Input: part model. Units: mm. Frame: model coordinates. A direction names the side the tool comes from. Coordinates: 2 decimals unless noted, no trailing zeros. Loops run counter-clockwise (first coordinate to the right, second up) from the corner with the lowest first, then second, coordinate; pieces in that order, holes last. Notation, with made-up numbers: (-39, 63.25) - (-4, 63.25) arc R9 ccw to (-4, 70.25) - close; hole circle Ø8 at (-3, -34.5). An arc over 180 degrees is marked (long way). Write item = value, one per line. Start each with the question number.
from build123d import *

# Parameters (mm, degrees)
F1_DEPTH    = 76.2
F2_T1_DEPTH = 369.824
F2_T3_DEPTH = 369.824


# Not quite as in the source:
# - a fillet or chamfer that OpenCascade refuses, or shapes differently, is made with other operations: its cross-section is extruded or revolved along the edge and cut away or added


with BuildPart() as f1:
    # F0 (on Right) → F1 (new body, symmetric)
    with BuildSketch(Plane.YZ):
        with BuildLine():
            Line((-304.8, 0), (0, 0))
            Line((0, 0), (304.8, 0))
            ThreePointArc((304.8, 0), (353.0430518596, 9.3618295777), (390.9983313803, 40.5777335736))
            Line((390.9983313803, 40.5777335736), (381.1075556217, 50.8))
            ThreePointArc((381.1075556217, 50.8), (346.1246462325, 27.304174222), (304.8, 19.05))
            Line((304.8, 19.05), (0, 19.05))
            Line((0, 19.05), (-304.8, 19.05))
            ThreePointArc((-304.8, 19.05), (-346.1246462325, 27.304174222), (-381.1075556217, 50.8))
            Line((-381.1075556217, 50.8), (-390.9983313803, 40.5777335736))
            ThreePointArc((-390.9983313803, 40.5777335736), (-353.0430518596, 9.3618295777), (-304.8, 0))
        make_face()
    extrude(amount=F1_DEPTH, both=True)

    # F2: fillet of radius 71.12 on 4 edges, made by hand

    # F2_s2 → F2_t1 (cut)
    with BuildSketch(Plane(origin=(0, -35.2534039099, -36.4349264406), x_dir=(1, 0, 0), z_dir=(0, -0.6953582507, -0.7186632752))):
        with BuildLine():
            ThreePointArc((5.08, 309.212203264), (55.369434278, 288.381637542), (76.2, 238.092203264))
            Line((76.2, 238.092203264), (76.2, 309.212203264))
            Line((76.2, 309.212203264), (5.08, 309.212203264))
        make_face()
        with BuildLine():
            ThreePointArc((-5.08, 309.212203264), (-55.369434278, 288.381637542), (-76.2, 238.092203264))
            Line((-76.2, 238.092203264), (-76.2, 309.212203264))
            Line((-76.2, 309.212203264), (-5.08, 309.212203264))
        make_face()
    extrude(amount=F2_T1_DEPTH, mode=Mode.SUBTRACT)

    # F2_s4 → F2_t3 (cut)
    with BuildSketch(Plane(origin=(0, 292.4135736338, -302.2138535277), x_dir=(1, 0, 0), z_dir=(0, -0.6953582507, 0.7186632752))):
        with BuildLine():
            ThreePointArc((5.08, 309.212203264), (55.369434278, 288.381637542), (76.2, 238.092203264))
            Line((76.2, 238.092203264), (76.2, 309.212203264))
            Line((76.2, 309.212203264), (5.08, 309.212203264))
        make_face()
        with BuildLine():
            ThreePointArc((-5.08, 309.212203264), (-55.369434278, 288.381637542), (-76.2, 238.092203264))
            Line((-76.2, 238.092203264), (-76.2, 309.212203264))
            Line((-76.2, 309.212203264), (-5.08, 309.212203264))
        make_face()
    extrude(amount=F2_T3_DEPTH, mode=Mode.SUBTRACT)


solid = f1.part
Item 1: Pull-direction query (Y, two-part tool) for faces 3 (the cylindrical face through (1.07, 337.84, 24.25)), 4 (the flat face through (-76.2, -5, 10)), 5 (the cylindrical face through (-54.81, 369.75, 33.38)); classes: pulls with the +Y half, pulls with the -Y half, needs draft (parallel to the pull), parting line crosses it, or undercut.
Item 2: Cut plane A-A on x = 59.5. Return loops of the section in (y, z), plus the area to 3 significant figures.
Item 3: Ray query, line 1 (Z direction, x = -49.5, y = -285); line 2 (Y direction, x = 41, z = 13); line 3 (Y direction, x = -7, z = 44). Return the intervals inside material, ascending.
Item 4: Pin query (flat end, axial travel): pin 1 (1 mm diameter, centred on x = 7, z = 17.5, fed in from -Y); pin 2 (10 mm diameter, centred on y = -183, z = 28, fed in from +X); pin 3 (10 mm diameter, centred on x = -50.5, y = -21, fed in from -Z); pin 4 (10 mm diameter, centred on x = 6.5, z = 7, fed in from -Y). Return the tip coordinate at first contact, or that it passes through.
Item 5: Cut plane B-B on y = -136.5. Return loops of the section in (x, z).
Item 6: Cut plane C-C on x = -46. Return loops of the section in (y, z).
Item 7: Access query for faces 1 (the flat face through (76.2, -5, 10)), 2 (the cylindrical face through (1.07, -336.71, 23.89)). Directions: +Z, -Z, +X, -X, +Y, -Y. A direction counts if a zero-diameter tool reaches every point of the face in a straight line with its end or side. Return the directions, or none.
Recorded:
q1.face_3 = undercut
q1.face_4 = needs draft
q1.face_5 = pulls with the +Y half
q2.outline = (-373.51, 22.22) arc R99.98 ccw to (-304.8, 0) - (304.8, 0) arc R99.98 ccw to (373.51, 22.22) - (361.15, 34.99) arc R107.57 cw to (304.8, 19.05) - (-304.8, 19.05) arc R107.57 cw to (-361.15, 34.99) - close
q2.area = 14,200 mm²
q3.line_1 = 0 to 19.05
q3.line_2 = -360.04 to 360.04
q3.line_3 = -387.65 to -373.69, 373.69 to 387.65
q4.pin_1 = -367.92
q4.pin_2 = through
q4.pin_3 = 0
q4.pin_4 = -358.25
q5.outline = (-76.2, 0) - (76.2, 0) - (76.2, 19.05) - (-76.2, 19.05) - close
q6.outline = (-382.62, 30.61) arc R99.98 ccw to (-304.8, 0) - (304.8, 0) arc R99.98 ccw to (382.62, 30.61) - (371.43, 42.17) arc R107.57 cw to (304.8, 19.05) - (-304.8, 19.05) arc R107.57 cw to (-371.43, 42.17) - close
q7.face_1 = +Z, -Z, +X, +Y, -Y
q7.face_2 = +Z, +X, -X
